Build history of the part. All positions in model axes, mm. A direction names the side the tool comes from. Round coordinates to 2 decimals unless told otherwise and drop trailing zeros. Write each loop counter-clockwise with the first axis right and the second up, starting at its lowest first coordinate (ties: lowest second). Pieces come first, ordered by that corner, then holes. Notation, with made-up numbers: (78, 12.5) -> (96, 12.5) arc R24 ccw to (96, 37.5) -> close; hole circle Ø10 at (-34, -2.5). An arc over 180 degrees is marked (long way). Answer in a Markdown table with one row per item.
```python
from build123d import *

# Parameters (mm, degrees)
SKETCH1_R           = 25.4
BOSS_EXTRUDE1_DEPTH = 6.35
SKETCH2_R           = 15.875
BOSS_EXTRUDE2_DEPTH = 9.525
SKETCH3_R           = 4.7625
CUT_EXTRUDE1_DEPTH  = 15.875
CUT_EXTRUDE2_DEPTH  = 6.35


with BuildPart() as part:
    # Sketch1 → Boss-Extrude1 (new body)
    with BuildSketch(Plane.XY):
        Circle(SKETCH1_R)
    extrude(amount=BOSS_EXTRUDE1_DEPTH)

    # Sketch2 → Boss-Extrude2 (add)
    with BuildSketch(Plane.XY.offset(6.35)):
        with Locations(Location((0, 0, 0), (0, 0, 180))):
            Circle(SKETCH2_R)
    extrude(amount=BOSS_EXTRUDE2_DEPTH)

    # Sketch3 → Cut-Extrude1 (cut)
    with BuildSketch(Plane.XY.offset(15.875)):
        Circle(SKETCH3_R)
    extrude(amount=-CUT_EXTRUDE1_DEPTH, mode=Mode.SUBTRACT)

    # Sketch4 → Cut-Extrude2 (cut)
    with BuildSketch(Plane(origin=(0, 0, 0), x_dir=(-1, 0, 0), z_dir=(0, 0, -1))):
        with BuildLine():
            Line((0, 25.4), (0, 23.368))
            ThreePointArc((0, 23.368), (23.368, 0), (0, -23.368))
            Line((0, -23.368), (0, -25.4))
            ThreePointArc((0, -25.4), (25.4, 0), (0, 25.4))
        make_face()
    extrude(amount=-CUT_EXTRUDE2_DEPTH, mode=Mode.SUBTRACT)


solid = part.part
```
Q1. Saw through at A-A on x = 4. Write the cut outline in (y, z) (3 decimals).
A:
| item | result |
|---|---|
| outline | (-25.083, 0) -> (-2.585, 0) -> (-2.585, 15.875) -> (-15.363, 15.875) -> (-15.363, 6.35) -> (-25.083, 6.35) -> close; (2.585, 0) -> (25.083, 0) -> (25.083, 6.35) -> (15.363, 6.35) -> (15.363, 15.875) -> (2.585, 15.875) -> close |
Q2. Wall check: line 1 (Y direction, x = 0, z = 9.5) (1 decimal); line 2 (Y direction, x = 2, z = 14.5); line 3 (Z direction, x = 7.5, y = 15). Give the ranges that are in metal, low to high. Write a range as [from, to].
A:
| item | result |
|---|---|
| line 1 | [-15.9, -4.8], [4.8, 15.9] |
| line 2 | [-15.75, -4.32], [4.32, 15.75] |
| line 3 | [0, 6.35] |
Q3. Two-plate mould, pull along X, no slides. Class faces 4 (the cylindrical face through (3.441, 15.497, 11.046)), 5 (the cylindrical face through (-23.362, 0.514, 3.131)), 6 (the cylindrical face through (-3.78, -2.9, 8.05)), 7 (the flat face through (6, 0, 0)): released by +X, released by -X, zero draft, split by the parting line, or undercut.
A:
| item | result |
|---|---|
| face 4 | split by the parting line |
| face 5 | released by -X |
| face 6 | undercut |
| face 7 | zero draft |
Q4. Saw through at D-D on y = -13. Write the cut outline in (x, z) (3 decimals), plus the area to 3 significant figures.
A:
| item | result |
|---|---|
| outline | (-19.418, 0) -> (21.821, 0) -> (21.821, 6.35) -> (9.111, 6.35) -> (9.111, 15.875) -> (-9.111, 15.875) -> (-9.111, 6.35) -> (-19.418, 6.35) -> close |
| area | 435 mm² |
Q5. Drop flat-ended pins along their axis: P1, Ø6, axis at y = -15.5, z = 7.5, coming from the -X side; P2, Ø3, axis at x = -4, z = 10.5, coming from the -Y side; P3, Ø2, axis at y = -24.5, z = 4, coming from the -X side. Give the stop position or say it passes through.
A:
| item | result |
|---|---|
| P1 | x = -19.6 |
| P2 | y = -15.68 |
| P3 | x = 0 |
Q6. Saw through at C-C on z = 1.5. Write the cut outline in (x, y) (1 decimal).
A:
| item | result |
|---|---|
| outline | (0, -25.4) arc R25.4 ccw to (0, 25.4) -> (0, 23.4) arc R23.4 ccw to (0, -23.4) -> close; hole circle Ø9.5 at (0, 0) |
Q7. Saw through at B-B on y = 1. Write the cut outline in (x, z) (3 decimals).
A:
| item | result |
|---|---|
| outline | (-23.347, 0) -> (-4.656, 0) -> (-4.656, 15.875) -> (-15.843, 15.875) -> (-15.843, 6.35) -> (-23.347, 6.35) -> close; (4.656, 0) -> (25.38, 0) -> (25.38, 6.35) -> (15.843, 6.35) -> (15.843, 15.875) -> (4.656, 15.875) -> close |
Q8. Which spindle directions (+Z, -Z, +X, -X, +Y, -Y) get a long thin tool onto all of the face, cutting with end or side? Do faces 1 (the flat face through (0, -24, 3)), 2 (the flat face through (12, -11, 6.35)), 3 (the flat face through (0, 24, 3)). Say none if no direction does.
A:
| item | result |
|---|---|
| face 1 | +Z, -Z, -X, -Y |
| face 2 | +Z |
| face 3 | +Z, -Z, -X, +Y |
